Verification items for the finished model (mm, model axes). A direction names the side the tool comes from. Give positions to 0.01 mm unless a question says otherwise; leave off trailing zeros. Order: outer loops, then holes, each group sorted by start corner. A loop starts at its lowest first (then second) coordinate and runs counter-clockwise, first axis right, second up. Notation, with made-up numbers: (35.25, 18) - (75.25, 18) arc R19 ccw to (75.25, 37) - close; hole circle Ø1 at (-21.75, 38). An arc over 180 degrees is marked (long way). Answer as a JSON object with one key per item and string values. Group by question number.
(1) Depth check by flat-ended pin: pin 1 Ø4 at (x, z) = (-63.5, 0) entering from +Y. Enter the tip coordinate at first touch or a pass-through.
(2) Access from +Z, -Z, +X, -X, +Y, -Y to the whole of each face (thin tool, end or side, straight path). Record for faces 5 (the face through (50.8, 3, -56)), 6 (the face through (-28.448, 3, -62)), 7 (the face through (-15.748, 3, 62)), 8 (the face through (-49, 3, -3.048)), 9 (the face through (49, 3, 15.748)).
(3) Thickness scan on line 1 (X direction, y = 3, z = -12.7); line 2 (X direction, y = 5.5, z = 42); line 3 (Z direction, x = -21, y = 4.25). Record the ranges inside material, lowest first.
(4) Section check B-B (x = -76.2). Count the separate pieces of the cut face and the enclosed holes in it, then the cut area to 3 significant figures.
(5) Section check A-A (z = 0). Record the boundary of the cut face in (x, y).
(6) Section check D-D (z = 39). Record the boundary of the cut face in (x, y).
(7) Mould release check, pull along Z, two halves, no side actions. Record for faces 1 (the face through (-66.542, 3.219, -11.118)), 2 (the face through (-13, 3, 63.5)), 3 (the face through (-25, 3, -63.5)), 4 (the face through (-22.352, 3, 62)): +Z half, -Z half, draft (parallel to the pull), parting line (faces both ways), or undercut.
```python
from build123d import *

# Parameters (mm, degrees)
SKETCH1_W           = 101.6
SKETCH1_H           = 127
BOSS_EXTRUDE1_DEPTH = 6.35
SKETCH2_W           = 6.604
SKETCH2_H           = 3.302
SKETCH2_W_2         = 3.429
SKETCH2_H_2         = 6.604
CUT_EXTRUDE1_DEPTH  = 82.567226875
SKETCH3_W           = 63.5
SKETCH3_H           = 127
SKETCH3_R           = 3.429
BOSS_EXTRUDE2_DEPTH = 6.35


with BuildPart() as part:
    # Sketch1 → Boss-Extrude1 (new body)
    with BuildSketch(Plane(origin=(0, 0, 0), x_dir=(1, 0, 0), z_dir=(0, 1, 0))):
        Rectangle(SKETCH1_W, SKETCH1_H)
    extrude(amount=BOSS_EXTRUDE1_DEPTH)

    # Sketch2 → Cut-Extrude1 (cut, through all)
    with BuildSketch(Plane(origin=(0, 6.35, 0), x_dir=(1, 0, 0), z_dir=(0, 1, 0))):
        with Locations((-31.75, -61.849)):
            Rectangle(SKETCH2_W, SKETCH2_H)
        with Locations((-19.05, -61.849)):
            Rectangle(SKETCH2_W, SKETCH2_H)
        with Locations((-6.35, -61.849)):
            Rectangle(SKETCH2_W, SKETCH2_H)
        with Locations((6.35, -61.849)):
            Rectangle(SKETCH2_W, SKETCH2_H)
        with Locations((19.05, -61.849)):
            Rectangle(SKETCH2_W, SKETCH2_H)
        with Locations((31.75, -61.849)):
            Rectangle(SKETCH2_W, SKETCH2_H)
        with Locations((31.75, 61.849)):
            Rectangle(SKETCH2_W, SKETCH2_H)
        with Locations((19.05, 61.849)):
            Rectangle(SKETCH2_W, SKETCH2_H)
        with Locations((6.35, 61.849)):
            Rectangle(SKETCH2_W, SKETCH2_H)
        with Locations((-6.35, 61.849)):
            Rectangle(SKETCH2_W, SKETCH2_H)
        with Locations((-19.05, 61.849)):
            Rectangle(SKETCH2_W, SKETCH2_H)
        with Locations((-31.75, 61.849)):
            Rectangle(SKETCH2_W, SKETCH2_H)
        with Locations((-49.0855, 31.75)):
            Rectangle(SKETCH2_W_2, SKETCH2_H_2)
        with Locations((-49.0855, 19.05)):
            Rectangle(SKETCH2_W_2, SKETCH2_H_2)
        with Locations((-49.0855, 6.35)):
            Rectangle(SKETCH2_W_2, SKETCH2_H_2)
        with Locations((-49.0855, -6.35)):
            Rectangle(SKETCH2_W_2, SKETCH2_H_2)
        with Locations((-49.0855, -19.05)):
            Rectangle(SKETCH2_W_2, SKETCH2_H_2)
        with Locations((-49.0855, -31.75)):
            Rectangle(SKETCH2_W_2, SKETCH2_H_2)
        with Locations((49.0855, -31.75)):
            Rectangle(SKETCH2_W_2, SKETCH2_H_2)
        with Locations((49.0855, -19.05)):
            Rectangle(SKETCH2_W_2, SKETCH2_H_2)
        with Locations((49.0855, -6.35)):
            Rectangle(SKETCH2_W_2, SKETCH2_H_2)
        with Locations((49.0855, 6.35)):
            Rectangle(SKETCH2_W_2, SKETCH2_H_2)
        with Locations((49.0855, 19.05)):
            Rectangle(SKETCH2_W_2, SKETCH2_H_2)
        with Locations((49.0855, 31.75)):
            Rectangle(SKETCH2_W_2, SKETCH2_H_2)
        with Locations((-49.0855, 44.45)):
            Rectangle(SKETCH2_W_2, SKETCH2_H_2)
        with Locations((-49.0855, -44.45)):
            Rectangle(SKETCH2_W_2, SKETCH2_H_2)
        with Locations((49.0855, -44.45)):
            Rectangle(SKETCH2_W_2, SKETCH2_H_2)
        with Locations((49.0855, 44.45)):
            Rectangle(SKETCH2_W_2, SKETCH2_H_2)
    extrude(amount=-CUT_EXTRUDE1_DEPTH, mode=Mode.SUBTRACT)

    # Sketch3 → Boss-Extrude2 (add)
    with BuildSketch(Plane(origin=(0, 6.35, 0), x_dir=(1, 0, 0), z_dir=(0, 1, 0))):
        with Locations((-82.55, 0)):
            Rectangle(SKETCH3_W, SKETCH3_H)
        with Locations(Location((-101.6, 50.8, 0), (0, 0, 270))):
            Circle(SKETCH3_R, mode=Mode.SUBTRACT)
        with Locations(Location((-88.9, 50.8, 0), (0, 0, 270))):
            Circle(SKETCH3_R, mode=Mode.SUBTRACT)
        with Locations(Location((-88.9, 38.1, 0), (0, 0, 270))):
            Circle(SKETCH3_R, mode=Mode.SUBTRACT)
        with Locations(Location((-101.6, 38.1, 0), (0, 0, 270))):
            Circle(SKETCH3_R, mode=Mode.SUBTRACT)
        with Locations(Location((-101.6, 25.4, 0), (0, 0, 270))):
            Circle(SKETCH3_R, mode=Mode.SUBTRACT)
        with Locations(Location((-88.9, 25.4, 0), (0, 0, 270))):
            Circle(SKETCH3_R, mode=Mode.SUBTRACT)
        with Locations(Location((-76.2, 50.8, 0), (0, 0, 270))):
            Circle(SKETCH3_R, mode=Mode.SUBTRACT)
        with Locations(Location((-63.5, 50.8, 0), (0, 0, 270))):
            Circle(SKETCH3_R, mode=Mode.SUBTRACT)
        with Locations(Location((-76.2, 38.1, 0), (0, 0, 270))):
            Circle(SKETCH3_R, mode=Mode.SUBTRACT)
        with Locations(Location((-63.5, 38.1, 0), (0, 0, 270))):
            Circle(SKETCH3_R, mode=Mode.SUBTRACT)
        with Locations(Location((-76.2, 25.4, 0), (0, 0, 270))):
            Circle(SKETCH3_R, mode=Mode.SUBTRACT)
        with Locations(Location((-63.5, 25.4, 0), (0, 0, 270))):
            Circle(SKETCH3_R, mode=Mode.SUBTRACT)
        with Locations(Location((-101.6, 12.7, 0), (0, 0, 270))):
            Circle(SKETCH3_R, mode=Mode.SUBTRACT)
        with Locations(Location((-88.9, 12.7, 0), (0, 0, 270))):
            Circle(SKETCH3_R, mode=Mode.SUBTRACT)
        with Locations(Location((-76.2, 12.7, 0), (0, 0, 270))):
            Circle(SKETCH3_R, mode=Mode.SUBTRACT)
        with Locations(Location((-63.5, 12.7, 0), (0, 0, 270))):
            Circle(SKETCH3_R, mode=Mode.SUBTRACT)
        with Locations(Location((-101.6, 0, 0), (0, 0, 270))):
            Circle(SKETCH3_R, mode=Mode.SUBTRACT)
        with Locations(Location((-88.9, 0, 0), (0, 0, 270))):
            Circle(SKETCH3_R, mode=Mode.SUBTRACT)
        with Locations(Location((-76.2, 0, 0), (0, 0, 270))):
            Circle(SKETCH3_R, mode=Mode.SUBTRACT)
        with Locations(Location((-63.5, 0, 0), (0, 0, 270))):
            Circle(SKETCH3_R, mode=Mode.SUBTRACT)
        with Locations(Location((-101.6, -12.7, 0), (0, 0, 270))):
            Circle(SKETCH3_R, mode=Mode.SUBTRACT)
        with Locations(Location((-88.9, -12.7, 0), (0, 0, 270))):
            Circle(SKETCH3_R, mode=Mode.SUBTRACT)
        with Locations(Location((-76.2, -12.7, 0), (0, 0, 270))):
            Circle(SKETCH3_R, mode=Mode.SUBTRACT)
        with Locations(Location((-63.5, -12.7, 0), (0, 0, 270))):
            Circle(SKETCH3_R, mode=Mode.SUBTRACT)
        with Locations(Location((-101.6, -25.4, 0), (0, 0, 270))):
            Circle(SKETCH3_R, mode=Mode.SUBTRACT)
        with Locations(Location((-88.9, -25.4, 0), (0, 0, 270))):
            Circle(SKETCH3_R, mode=Mode.SUBTRACT)
        with Locations(Location((-76.2, -25.4, 0), (0, 0, 270))):
            Circle(SKETCH3_R, mode=Mode.SUBTRACT)
        with Locations(Location((-63.5, -25.4, 0), (0, 0, 270))):
            Circle(SKETCH3_R, mode=Mode.SUBTRACT)
        with Locations(Location((-101.6, -38.1, 0), (0, 0, 270))):
            Circle(SKETCH3_R, mode=Mode.SUBTRACT)
        with Locations(Location((-88.9, -38.1, 0), (0, 0, 270))):
            Circle(SKETCH3_R, mode=Mode.SUBTRACT)
        with Locations(Location((-76.2, -38.1, 0), (0, 0, 270))):
            Circle(SKETCH3_R, mode=Mode.SUBTRACT)
        with Locations(Location((-63.5, -38.1, 0), (0, 0, 270))):
            Circle(SKETCH3_R, mode=Mode.SUBTRACT)
        with Locations(Location((-101.6, -50.8, 0), (0, 0, 270))):
            Circle(SKETCH3_R, mode=Mode.SUBTRACT)
        with Locations(Location((-88.9, -50.8, 0), (0, 0, 270))):
            Circle(SKETCH3_R, mode=Mode.SUBTRACT)
        with Locations(Location((-76.2, -50.8, 0), (0, 0, 270))):
            Circle(SKETCH3_R, mode=Mode.SUBTRACT)
        with Locations(Location((-63.5, -50.8, 0), (0, 0, 270))):
            Circle(SKETCH3_R, mode=Mode.SUBTRACT)
    extrude(amount=-BOSS_EXTRUDE2_DEPTH)


solid = part.part
```
Solutions:
{
 "1": {"pin 1": "passes through"},
 "2": {"face 5": "+Z, -Z, +X, +Y, -Y", "face 6": "-Z, +Y, -Y", "face 7": "+Z, +Y, -Y", "face 8": "+Y, -Y", "face 9": "+X, +Y, -Y"},
 "3": {"line 1": "x = -114.3 to -105.03, -98.17 to -92.33, -85.47 to -79.63, -72.77 to -66.93, -60.07 to 50.8", "line 2": "x = -114.3 to -50.8, -47.37 to 47.37", "line 3": "z = -60.2 to 60.2"},
 "4": {"separate pieces": "10", "enclosed holes": "0", "area": "415 mm2"},
 "5": {"outline": "(-114.3, 0) - (-105.03, 0) - (-105.03, 6.35) - (-114.3, 6.35) - close; (-98.17, 0) - (-92.33, 0) - (-92.33, 6.35) - (-98.17, 6.35) - close; (-85.47, 0) - (-79.63, 0) - (-79.63, 6.35) - (-85.47, 6.35) - close; (-72.77, 0) - (-66.93, 0) - (-66.93, 6.35) - (-72.77, 6.35) - close; (-60.07, 0) - (50.8, 0) - (50.8, 6.35) - (-60.07, 6.35) - close"},
 "6": {"outline": "(-114.3, 0) - (-104.91, 0) - (-104.91, 6.35) - (-114.3, 6.35) - close; (-98.29, 0) - (-92.21, 0) - (-92.21, 6.35) - (-98.29, 6.35) - close; (-85.59, 0) - (-79.51, 0) - (-79.51, 6.35) - (-85.59, 6.35) - close; (-72.89, 0) - (-66.81, 0) - (-66.81, 6.35) - (-72.89, 6.35) - close; (-60.19, 0) - (50.8, 0) - (50.8, 6.35) - (-60.19, 6.35) - close"},
 "7": {"face 1": "undercut", "face 2": "+Z half", "face 3": "-Z half", "face 4": "draft"}
}
